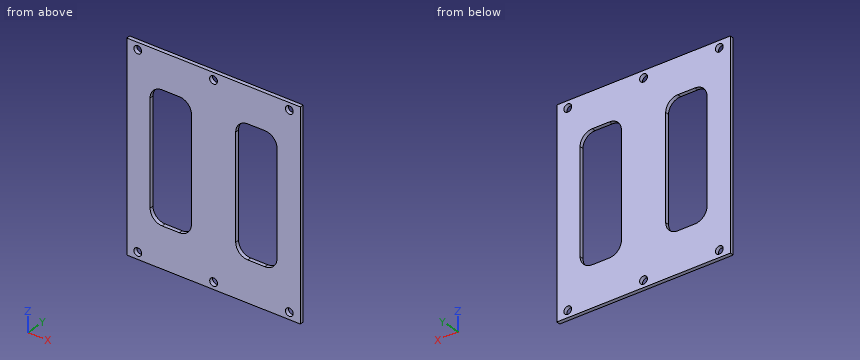
```python
from build123d import *

# Parameters (mm, degrees)
F0_W     = 72.7456
F0_H     = 85.09
F0_R     = 1.6383
F0_W_2   = 17.3228
F0_H_2   = 53.34
F1_DEPTH = 1.5875
F2_R     = 5.08


with BuildPart() as f1:
    # F0 (on Front) → F1 (new body)
    with BuildSketch(Plane.XZ):
        with Locations((0, 6.819942)):
            Rectangle(F0_W, F0_H)
        with Locations((-31.75, -32.804058)):
            Circle(F0_R, mode=Mode.SUBTRACT)
        with Locations((0.020847, -32.804058)):
            Circle(F0_R, mode=Mode.SUBTRACT)
        with Locations((31.75, -32.804058)):
            Circle(F0_R, mode=Mode.SUBTRACT)
        with Locations((-17.931937, 7.867827)):
            Rectangle(F0_W_2, F0_H_2, mode=Mode.SUBTRACT)
        with Locations((-31.75, 46.443942)):
            Circle(F0_R, mode=Mode.SUBTRACT)
        with Locations((0, 46.443942)):
            Circle(F0_R, mode=Mode.SUBTRACT)
        with Locations((17.931937, 7.867827)):
            Rectangle(F0_W_2, F0_H_2, mode=Mode.SUBTRACT)
        with Locations((31.75, 46.443942)):
            Circle(F0_R, mode=Mode.SUBTRACT)
    extrude(amount=F1_DEPTH)

    # F2
    f2_edges = [f1.edges().sort_by_distance(p)[0] for p in [
        (-26.593337, -0.79375, 34.537827),
        (-9.270537, -0.79375, 34.537827),
        (26.593337, -0.79375, -18.802173),
        (9.270537, -0.79375, -18.802173),
        (9.270537, -0.79375, 34.537827),
        (26.593337, -0.79375, 34.537827),
        (-9.270537, -0.79375, -18.802173),
        (-26.593337, -0.79375, -18.802173),
    ]]
    fillet(f2_edges, radius=F2_R)


solid = f1.part
```
The model under review builds one solid part; all positions refer to its coordinate system, in mm. Round coordinates to 2 decimals unless told otherwise and drop trailing zeros. Loops run counter-clockwise (first coordinate to the right, second up) from the corner with the lowest first, then second, coordinate; pieces in that order, holes last. Notation, with made-up numbers: M 87,48.25 L 102,48.25 A16 cw 102,62.25 Z; hole C 53.25,3 d4. An arc over 180 degrees is marked long. Put each result on its own line as item: value.
Q1. To check wall thickness, follow L1, parallel to X at y = -0.1, z = 1; L2, parallel to Z at x = 19, y = -0.8; L3, parallel to Z at x = 0, y = -0.4. State the ranges of each line that lie inside material, in increasing order.
Result set:
L1: x = -36.37 to -26.59, -9.27 to 9.27, 26.59 to 36.37
L2: z = -35.73 to -18.8, 34.54 to 49.36
L3: z = -35.73 to -34.44, -31.17 to 44.81, 48.08 to 49.36
Q2. Consider section D-D, the plane x = 23. Give the boundary of the cut face in (y, z), then the cut area to 3 significant figures.
Result set:
outline: M -1.59,-35.73 L 0,-35.73 L 0,-18.58 L -1.59,-18.58 Z; M -1.59,34.32 L 0,34.32 L 0,49.36 L -1.59,49.36 Z
area: 51.1 mm²
Q3. For pin 1 (8 mm diameter, centred on x = 26, z = 16.5, fed in from +Y), flat-tipped, find the tip position at first contact; note if it passes through.
Result set:
pin 1: stops at y = 0
Q4. Consider section C-C, the plane y = -0.55. Count the separate pieces of the cut face and the enclosed holes in it, then the cut area to 3 significant figures.
Result set:
separate pieces: 1
enclosed holes: 8
area: 4,340 mm²
Q5. Consider section B-B, the plane x = 31.75. Give the boundary of the cut face in (y, z), then the cut area to 3 significant figures.
Result set:
outline: M -1.59,-35.73 L 0,-35.73 L 0,-34.44 L -1.59,-34.44 Z; M -1.59,-31.17 L 0,-31.17 L 0,44.81 L -1.59,44.81 Z; M -1.59,48.08 L 0,48.08 L 0,49.36 L -1.59,49.36 Z
area: 125 mm²
Q6. Consider section A-A, the plane z = 28. Give the boundary of the cut face in (x, y), then the cut area to 3 significant figures.
Result set:
outline: M -36.37,-1.59 L -26.59,-1.59 L -26.59,0 L -36.37,0 Z; M -9.27,-1.59 L 9.27,-1.59 L 9.27,0 L -9.27,0 Z; M 26.59,-1.59 L 36.37,-1.59 L 36.37,0 L 26.59,0 Z
area: 60.5 mm²
